Build history of the part. All positions in model axes, mm. Coordinates: 2 decimals unless noted, no trailing zeros. Write each loop counter-clockwise with the first axis right and the second up, starting at its lowest first coordinate (ties: lowest second). Pieces come first, ordered by that corner, then holes. Notation, with made-up numbers: M -18,34 L 26,34 A13 cw 26,47 Z; hole C -16.75,-9 d2. An arc over 180 degrees is marked long. Use CSV: the item, a comma, the result in double quotes. Start each with the question number.
```python
from build123d import *

# Parameters (mm, degrees)
SKETCH1_W           = 110
SKETCH1_H           = 100
BOSS_EXTRUDE1_DEPTH = 2
FILLET2_R           = 40
SKETCH6_R           = 4
SKETCH6_W           = 40
SKETCH6_H           = 20
CUT_EXTRUDE4_DEPTH  = 3
SKETCH7_R           = 0.75
SKETCH7_R_2         = 3
CUT_EXTRUDE7_DEPTH  = 10
SKETCH8_R           = 0.75
CUT_EXTRUDE8_DEPTH  = 10


with BuildPart() as part:
    # Sketch1 → Boss-Extrude1 (new body)
    with BuildSketch(Plane.XY):
        with BuildLine():
            Line((-55, 50), (-55, -50))
            ThreePointArc((-55, -50), (-75, 0), (-55, 50))
        make_face()
        Rectangle(SKETCH1_W, SKETCH1_H)
        with BuildLine():
            ThreePointArc((55, 50), (75, 0), (55, -50))
            Line((55, -50), (55, 50))
        make_face()
    extrude(amount=BOSS_EXTRUDE1_DEPTH)

    # Fillet2
    fillet2_edges = [part.edges().sort_by_distance(p)[0] for p in [
        (-55, 50, 1),
        (55, 50, 1),
        (55, -50, 1),
        (-55, -50, 1),
    ]]
    fillet(fillet2_edges, radius=FILLET2_R)

    # Sketch6 → Cut-Extrude4 (cut)
    with BuildSketch(Plane.XY.offset(2)):
        with Locations((-24, -19)):
            Circle(SKETCH6_R)
        with Locations((-40, 0)):
            Rectangle(SKETCH6_W, SKETCH6_H)
    extrude(amount=-CUT_EXTRUDE4_DEPTH, mode=Mode.SUBTRACT)

    # Sketch7 → Cut-Extrude7 (cut)
    with BuildSketch(Plane.XY.offset(2)):
        with Locations((-7, 38.5)):
            Circle(SKETCH7_R)
        with Locations((55, 38.5)):
            Circle(SKETCH7_R)
        with Locations((55, -38.5)):
            Circle(SKETCH7_R)
        with Locations((-7, -38.5)):
            Circle(SKETCH7_R)
        with Locations((59, 16)):
            Circle(SKETCH7_R_2)
        with Locations((59, -16)):
            Circle(SKETCH7_R_2)
        with Locations((59, 0)):
            Circle(SKETCH7_R_2)
    extrude(amount=-CUT_EXTRUDE7_DEPTH, mode=Mode.SUBTRACT)

    # Sketch8 → Cut-Extrude8 (cut)
    with BuildSketch(Plane.XY.offset(2)):
        with Locations((-50, 37.5)):
            Circle(SKETCH8_R)
        with Locations((50, 37.5)):
            Circle(SKETCH8_R)
        with Locations((50, -37.5)):
            Circle(SKETCH8_R)
        with Locations((-50, -37.5)):
            Circle(SKETCH8_R)
    extrude(amount=-CUT_EXTRUDE8_DEPTH, mode=Mode.SUBTRACT)


solid = part.part
```
1. Drill centre lines: line 1 along Y through (x, z) = (-24, 0.5); line 2 along Y through (x, z) = (-7, 0.6); line 3 along X through (y, z) = (37.5, 0.7). Where is each one in solid material? Low to high. Write a range as from..to.
2. Pull direction Y, two halves, no side cores. Call faces 1 (the cylindrical face through (57.241, -42.136, 1.014)), 2 (the flat face through (1, 1, 2)), 3 (the cylindrical face through (-75, 0, 1)), 4 (the cylindrical face through (56, 0, 1)): pulls with the +Y half, pulls with the -Y half, needs draft (parallel to the pull), parting line crosses it, or undercut.
3. Slice it at B-B (x = -35). List the corners of the cut face in (y, z), and give its area (3 significant figures).
4. Slice it at C-C (y = 1.5). List the corners of the cut face in (x, z), and give its area (3 significant figures).
5. Slice it at D-D (x = 59). List the corners of the cut face in (y, z).
6. Slice it at A-A (z = 1.4). Count the separate pieces of the cut face and the enclosed holes in it, and give its area (3 significant figures).
7. Flat gauge pins, fed straight in: pin 1 (0.6 mm diameter, centred on x = -40.5, z = 1, fed in from -Y); pin 2 (9 mm diameter, centred on x = -24, y = -19, fed in from +Z). Where does each tip first touch, or does it go through?
Established:
1,line 1,"y = -50..-23, -15..-10, 10..50"
1,line 2,"y = -50..-39.25, -37.75..37.75, 39.25..50"
1,line 3,"x = -62.47..-50.75, -49.25..49.25, 50.75..62.47"
2,face 1,"pulls with the -Y half"
2,face 2,"needs draft"
2,face 3,"parting line crosses it"
2,face 4,"undercut"
3,outline,"M -49.97,0 L -10,0 L -10,2 L -49.97,2 Z; M 10,0 L 49.97,0 L 49.97,2 L 10,2 Z"
3,area,"160 mm2"
4,outline,"M -74.98,0 L -60,0 L -60,2 L -74.98,2 Z; M -20,0 L 56.4,0 L 56.4,2 L -20,2 Z; M 61.6,0 L 74.98,0 L 74.98,2 L 61.6,2 Z"
4,area,"210 mm2"
5,outline,"M -40.75,0 L -19,0 L -19,2 L -40.75,2 Z; M -13,0 L -3,0 L -3,2 L -13,2 Z; M 3,0 L 13,0 L 13,2 L 3,2 Z; M 19,0 L 40.75,0 L 40.75,2 L 19,2 Z"
6,separate pieces,"1"
6,enclosed holes,"13"
6,area,"12,400 mm2"
7,pin 1,"stops at y = -49.42"
7,pin 2,"stops at z = 2"
